The figure shows three views and two pictorial views of one solid part (mm, origin at its lowest corner). Answer the questions. Round coordinates to 2 decimals unless told otherwise and drop trailing zeros. Loops run counter-clockwise (first coordinate to the right, second up) from the corner with the lowest first, then second, coordinate; pieces in that order, holes last. Notation, with made-up numbers: (-26.75, -31.5) -> (26.25, -31.5) arc R23 ccw to (26.25, -15.5) -> close; hole circle Ø6 at (-24, -31.5). An arc over 180 degrees is marked (long way). Put each result on its own line as item: value.
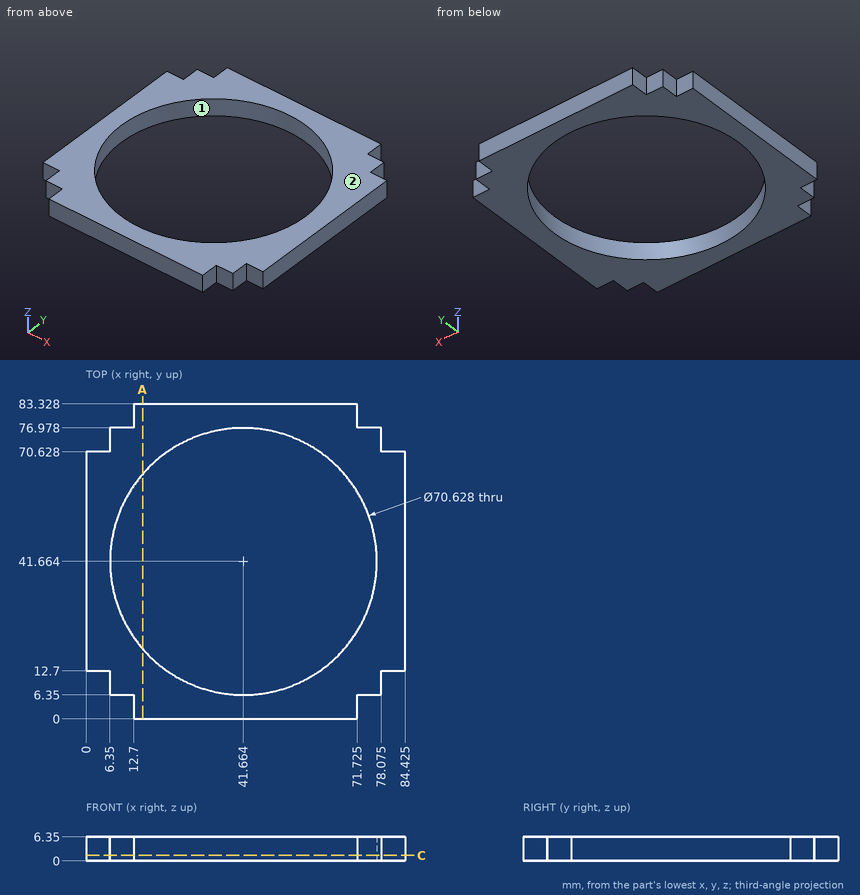
Item 1: For a pull along X with two mould halves and no side action, classify the marked faces 1 and 2 as pulls with the +X half, pulls with the -X half, needs draft (parallel to the pull), parting line crosses it, or undercut.
Derived:
face 1: undercut
face 2: needs draft
Item 2: The part is cut by section A-A (x = 15). Determine the outline of the cut face in (y, z).
Derived:
outline: (0, 0) -> (18.51, 0) -> (18.51, 6.35) -> (0, 6.35) -> close; (64.82, 0) -> (83.33, 0) -> (83.33, 6.35) -> (64.82, 6.35) -> close
Item 3: The part is cut by section C-C (z = 1.5). Determine the outline of the cut face in (x, y) (3 decimals), then the cut area to 3 significant figures.
Derived:
outline: (0, 12.7) -> (6.35, 12.7) -> (6.35, 6.35) -> (12.7, 6.35) -> (12.7, 0) -> (71.725, 0) -> (71.725, 6.35) -> (78.075, 6.35) -> (78.075, 12.7) -> (84.425, 12.7) -> (84.425, 70.628) -> (78.075, 70.628) -> (78.075, 76.978) -> (71.725, 76.978) -> (71.725, 83.328) -> (12.7, 83.328) -> (12.7, 76.978) -> (6.35, 76.978) -> (6.35, 70.628) -> (0, 70.628) -> close; hole circle Ø70.628 at (41.664, 41.664)
area: 2,630 mm^2
Item 4: Flat-ended cylindrical pins translate along their axes: pin 1 Ø3 at (x, z) = (4.5, 2) entering from +Y; pin 2 Ø3 at (y, z) = (79, 3) entering from -X; pin 3 Ø3 at (x, z) = (73.5, 4.5) entering from +Y. Find the tip coordinate at first contact, or state that the pin passes through.
Derived:
pin 1: stops at y = 70.63
pin 2: stops at x = 12.7
pin 3: stops at y = 76.98
Item 5: Find the intervals of material crossed by line 1 along Y through (x, z) = (69, 2.75); line 2 along Y through (x, z) = (34, 1); line 3 along X through (y, z) = (20.5, 3.25) (1 decimal), in increasing order.
Derived:
line 1: y = 0 to 19.31, 64.02 to 83.33
line 2: y = 0 to 7.19, 76.14 to 83.33
line 3: x = 0 to 13.4, 69.9 to 84.4
